Autodesk Fusion 360 part; units mm, degrees
sketch "Sketch1" plane through (0, 0, 0) normal (0, 0, 1) x (1, 0, 0)
  circle A0 centre (0, 0) radius 6
  line L0 (0, 0) -> (0, 5) construction
  line L1 (0, 5) -> (3.3166, 5)
  line L2 (0, 5) -> (-3.3166, 5)
  line L3 (20, 0) -> (2.5, 0)
  line L4 (0, -5) -> (3.3166, -5)
  line L5 (0, -5) -> (-3.3166, -5)
  circle A1 centre (0, 0) radius 2.5
  circle A2 centre (0, 0) radius 3.9 construction
  line L6 (-3.9, 0) -> (-3.9, 1)
  line L7 (-3.9, 1) -> (-4.1, 1)
  line L8 (-4.1, 1) -> (-4.1, -1)
  line L9 (-4.1, -1) -> (-3.9, -1)
  line L10 (-3.9, -1) -> (-3.9, 0)
  line L11 (4.1, 1) -> (4.1, -1)
  line L12 (3.9, 0) -> (3.9, 1)
  line L13 (3.9, 1) -> (4.1, 1)
  line L14 (3.9, -1) -> (3.9, 0)
  line L15 (4.1, -1) -> (3.9, -1)
  line L16 (6, 0) -> (6, 5)
  line L17 (6, 5) -> (-6, 5)
  line L18 (-6, 5) -> (-6, -5)
  line L19 (-6, -5) -> (6, -5)
  line L20 (6, -5) -> (6, 0)
  dimension "d1" = 12
  dimension "d2" = 5
  dimension "d5" = 5
  dimension "d8" = 7.8
  dimension "d9" = 1
  dimension "d10" = 0.2
  dimension "d11" = 2
  dimension "d12" = 0.2
  dimension "d15" = 5
  dimension "d16" = 12
  dimension "d17" = 10
  dimension "d18" = 12
extrude "Extrude1" add sketch "Sketch1" along normal blind 15 contours A0 L1 L2 L4 L5 L17 L19 | A1 | L3 L11 L14 L15 | L3 L11 L12 L13 | L6 L7 L8 L9 L10
extrude "Extrude2" add sketch "Sketch1" against normal blind 1.7 contours A1
extrude "Extrude3" add sketch "Sketch1" against normal blind 3 contours L3 L11 L14 L15 | L3 L11 L12 L13 | L6 L7 L8 L9 L10
extrude "Extrude4" add sketch "Sketch1" along normal blind 18 from surface at 15 contours A0 L1 L2 L4 L5 L17 L19 | A0 L19 L20 | A1 | L3 L11 L14 L15 | L3 L11 L12 L13 | A0 L16 L17 | A0 L17 L18 | A0 L18 L19 | L6 L7 L8 L9 L10
sketch "Sketch2" plane through (0, 5, 0) normal (0, 1, 0) x (-1, 0, 0)
  line L0 (-15, 0) -> (-15, 5)
  line L1 (-15, 5) -> (-33, 5)
  line L2 (-33, 5) -> (-33, -5)
  line L3 (-33, -5) -> (-15, -5)
  line L4 (-15, -5) -> (-15, 0)
  line L5 (-15, 0) -> (-31, 0) construction
  line L6 (-31, 0) -> (-29.5, 0) construction
  circle A0 centre (-29.5, 0) radius 1.5
  line L7 (-3.3166, 0) -> (3.3166, 0)
  line L8 (3.3166, 0) -> (3.3166, 15)
  line L9 (3.3166, 15) -> (6, 15)
  line L10 (6, 15) -> (6, 33)
  line L11 (6, 33) -> (-6, 33)
  line L12 (-6, 33) -> (-6, 15)
  line L13 (-6, 15) -> (-3.3166, 15)
  line L14 (-3.3166, 15) -> (-3.3166, 0)
  line L15 (3.3166, 15) -> (-3.3166, 15)
  line L16 (0, 15) -> (0, 31) construction
  line L17 (0, 31) -> (0, 29.5) construction
  circle A1 centre (0, 29.5) radius 1.5
  dimension "d22" = 16
  dimension "d23" = 1.5
  dimension "d24" = 3
  dimension "d25" = 16
  dimension "d26" = 1.5
  dimension "d27" = 3
extrude "Extrude5" add sketch "Sketch2" along normal blind 8 contours A1
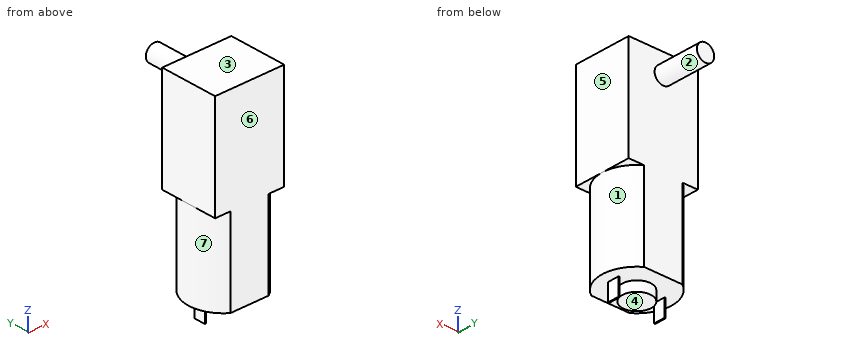
Design review of the part built by this model. Coordinates are the model's own, in mm. Face numbers are marked on the shaded views. A direction names the side the tool comes from. Round coordinates to 2 decimals unless told otherwise and drop trailing zeros. Write each loop counter-clockwise with the first axis right and the second up, starting at its lowest first coordinate (ties: lowest second). Pieces come first, ordered by that corner, then holes.
Item 1: Wall thickness on L1, parallel to Y at x = 2.75, z = 28.5; L2, parallel to Z at x = -4, y = -3.75; L3, parallel to Z at x = 4.5, y = 4.5: over which ranges is each line inside the solid? List them lowest first.
Item 2: For pin 1 Ø1.3 at (x, y) = (-4.5, -3) entering from -Z; pin 2 Ø0.6 at (y, z) = (0.5, -2) entering from +X; pin 3 Ø4 at (x, y) = (0, -1) entering from -Z; pin 4 Ø6 at (y, z) = (9.5, 6.5) entering from -X (3 decimals), all flat-tipped, find the tip position at first contact; note any pin that passes through.
Item 3: Consider section C-C on y = 3.5. Give the boundary of the cut face in (x, z), and give its area (3 significant figures).
Item 4: For the marked faces 1, 2 and 3, list the 3-axis set-ups (+Z, -Z, +X, -X, +Y, -Y) from which the entire face can be reached by the end or side of a thin tool; tool diameter is ignored.
Item 5: Draft analysis for pull direction X (two halves, no side actions). For the marked faces 4, 5, 6 and 7, state which applies: released by +X, released by -X, zero draft, split by the parting line, or undercut.
Item 6: Consider section B-B on x = 0. Give the boundary of the cut face in (y, z).
Item 7: Consider section D-D on z = 9.5. Give the boundary of the cut face in (x, y), and give its area (3 significant figures).
Item 8: Consider section A-A on z = 29.5. Give the boundary of the cut face in (x, y).
Check values:
1. L1: y = -5 to 5
1. L2: z = 0 to 33
1. L3: z = 15 to 33
2. pin 1: stops at z = 0
2. pin 2: stops at x = 4.1
2. pin 3: stops at z = -1.7
2. pin 4: passes through
3. outline: (-6, 15) - (-4.87, 15) - (-4.87, 0) - (4.87, 0) - (4.87, 15) - (6, 15) - (6, 33) - (-6, 33) - close
3. area: 362 mm2
4. face 1: -Z, +X
4. face 2: +Y
4. face 3: +Z, +X, -X, +Y, -Y
5. face 4: undercut
5. face 5: released by +X
5. face 6: zero draft
5. face 7: released by -X
6. outline: (-5, 0) - (-2.5, 0) - (-2.5, -1.7) - (2.5, -1.7) - (2.5, 0) - (5, 0) - (5, 28) - (13, 28) - (13, 31) - (5, 31) - (5, 33) - (-5, 33) - close
7. outline: (-3.32, -5) - (3.32, -5) arc R6 ccw to (3.32, 5) - (-3.32, 5) arc R6 ccw to start
7. area: 104 mm2
8. outline: (-6, -5) - (6, -5) - (6, 5) - (1.5, 5) - (1.5, 13) - (-1.5, 13) - (-1.5, 5) - (-6, 5) - close
